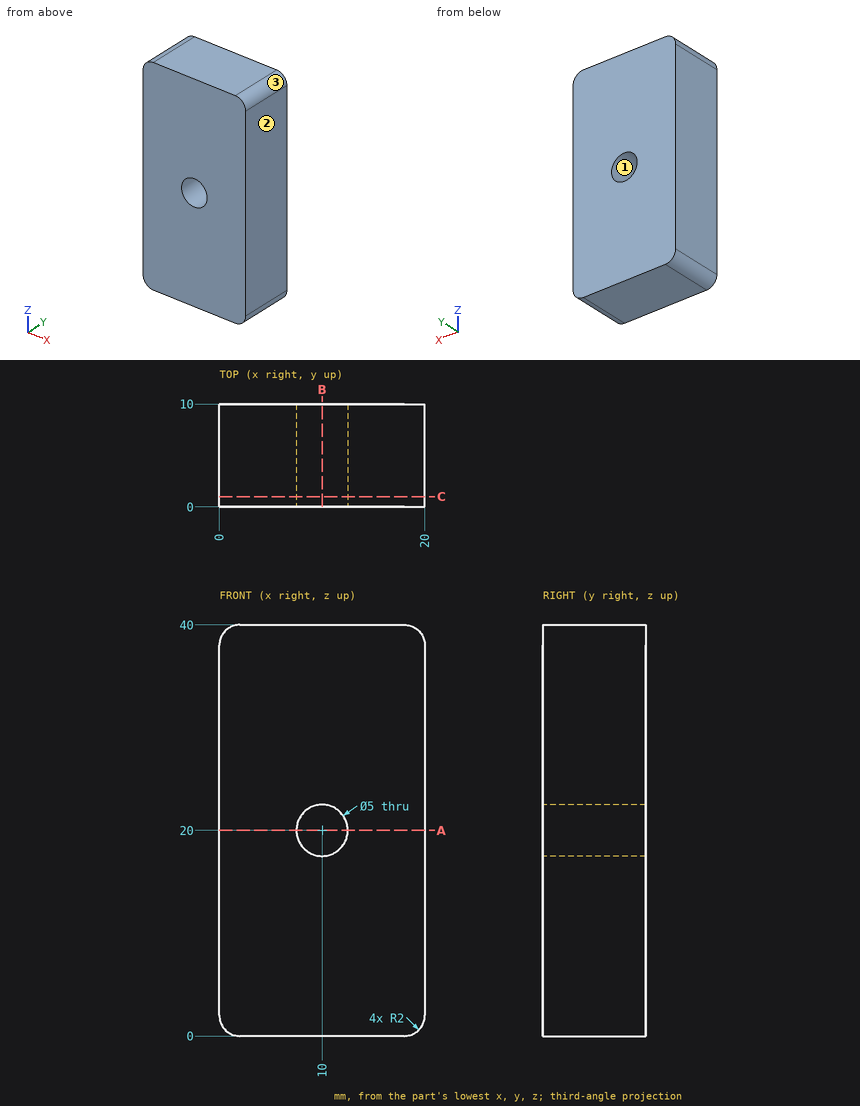
Geometry: see drawing. Coordinates: mm, zero at the bounding-box minimum. Coordinates: 2 decimals unless noted, no trailing zeros. Order: outer loops, then holes, each group sorted by start corner. A loop starts at its lowest first (then second) coordinate and runs counter-clockwise, first axis right, second up. Notation, with made-up numbers: (-21, 6) -> (-17, 6) arc R31 ccw to (-17, 43) -> close; hole circle Ø10 at (76, -4). An arc over 180 degrees is marked (long way). Write each question's results on one line, items separated by ' | '. Start each with the question number.
1) Cut plane B-B, the plane x = 10. Output: boundary loops of the cut face in (y, z), and give its area (3 significant figures).
2) Cut plane C-C, the plane y = 1. Output: boundary loops of the cut face in (x, z).
3) Cut plane A-A, the plane z = 20. Output: boundary loops of the cut face in (x, y), and give its area (3 significant figures).
4) Material intervals for line 1 along X through (y, z) = (7.5, 20); line 2 along Z through (x, y) = (10, 5.5); line 3 along Z through (x, y) = (9, 5), sorted ascending.
5) Mould query, pull axis Z, two halves, no side actions, for the marked faces 1, 2 and 3. Classes: released by +Z, released by -Z, zero draft, split by the parting line, or undercut.
Checks:
1) outline: (0, 0) -> (10, 0) -> (10, 17.5) -> (0, 17.5) -> close; (0, 22.5) -> (10, 22.5) -> (10, 40) -> (0, 40) -> close | area: 350 mm^2
2) outline: (0, 2) arc R2 ccw to (2, 0) -> (18, 0) arc R2 ccw to (20, 2) -> (20, 38) arc R2 ccw to (18, 40) -> (2, 40) arc R2 ccw to (0, 38) -> close; hole circle Ø5 at (10, 20)
3) outline: (0, 0) -> (7.5, 0) -> (7.5, 10) -> (0, 10) -> close; (12.5, 0) -> (20, 0) -> (20, 10) -> (12.5, 10) -> close | area: 150 mm^2
4) line 1: 0 to 7.5, 12.5 to 20 | line 2: 0 to 17.5, 22.5 to 40 | line 3: 0 to 17.71, 22.29 to 40
5) face 1: undercut | face 2: zero draft | face 3: released by +Z
